Input: dimensioned drawing with shaded views. Units: mm. Origin: part minimum x, y, z. A direction names the side the tool comes from. Round coordinates to 2 decimals unless told otherwise and drop trailing zeros. Loops run counter-clockwise (first coordinate to the right, second up) from the corner with the lowest first, then second, coordinate; pieces in that order, holes last.
Item 1: Access query for the marked faces 1, 2, 3 and 4. Directions: +Z, -Z, +X, -X, +Y, -Y. A direction counts if a zero-diameter tool reaches every point of the face in a straight line with its end or side. Return the directions, or none.
Item 2: Section query A-A on y = 16. Return loops of the section in (x, z).
Item 3: Section query B-B on x = 98. Return loops of the section in (y, z).
Item 4: Pull-direction query (X, two-part tool) for the marked faces 5, 6 and 7; classes: released by +X, released by -X, zero draft, split by the parting line, or undercut.
Item 5: First-contact query: P1, Ø11, axis at y = 19.5, z = 47.5, coming from the +X side; P2, Ø8, axis at y = 41, z = 14.5, coming from the +X side; P3, Ø22, axis at x = 17.5, z = 16.5, coming from the -Y side. Flat tips, straight axial feed; report the tip coordinate or a pass-through.
Item 6: Section query C-C on x = 45.5. Return loops of the section in (y, z), then the cut area to 4 significant figures.
Item 7: Section query D-D on z = 32. Return loops of the section in (x, y), then the cut area to 3 significant figures.
Item 8: Ray query, L1, parallel to Z at x = 76, y = 57.5; L2, parallel to X at y = 26.5, z = 46.5; L3, parallel to Y at x = 87, z = 22. Return the intervals inside material, ascending.
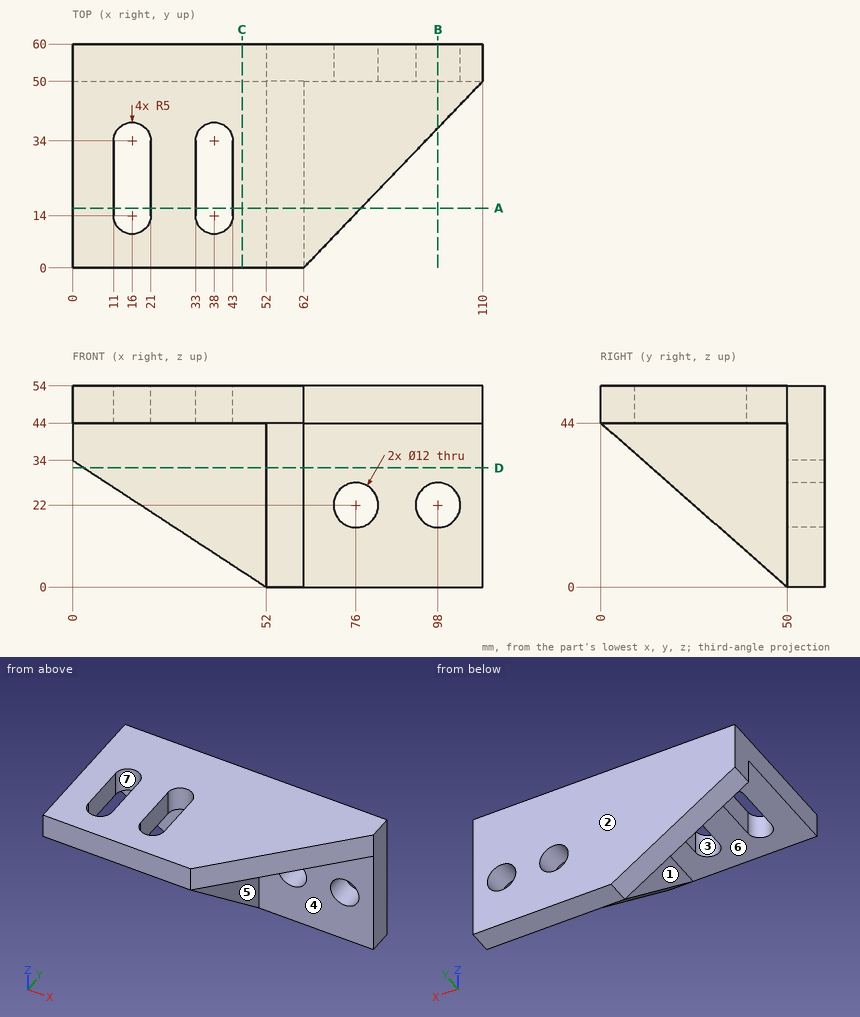
Data:
1. face 1: -Z, -X, -Y
1. face 2: +Z, -Z, +X, -X, +Y
1. face 3: +Z, -Z
1. face 4: -Z, +X, -Y
2. outline: (0, 44) - (11, 44) - (11, 54) - (0, 54) - close; (21, 44) - (33, 44) - (33, 54) - (21, 54) - close; (43, 44) - (52, 44) - (52, 29.92) - (62, 29.92) - (62, 44) - (77.36, 44) - (77.36, 54) - (43, 54) - close
3. outline: (37.5, 44) - (50, 44) - (50, 28) - (60, 28) - (60, 54) - (37.5, 54) - close; (50, 0) - (60, 0) - (60, 16) - (50, 16) - close
4. face 5: released by +X
4. face 6: zero draft
4. face 7: undercut
5. P1: stops at x = 86
5. P2: stops at x = 62
5. P3: stops at y = 50
6. outline: (0, 44) - (50, 44) - (50, 4.25) - (60, 4.25) - (60, 54) - (0, 54) - close
6. area: 997.5 mm2
7. outline: (3.06, 50) - (52, 50) - (52, 13.64) - (62, 13.64) - (62, 50) - (110, 50) - (110, 60) - (3.06, 60) - close
7. area: 1,430 mm2
8. L1: z = 0 to 16, 28 to 54
8. L2: x = 0 to 11, 21 to 33, 43 to 87.44
8. L3: y = 50 to 60
